from build123d import *

# Parameters (mm, degrees)
F1_DEPTH   = 25
F1_FACE_W  = 5
F1_FACE_H  = 25
F1_FACE1_W = 25
F1_FACE1_H = 25


with BuildPart() as f1:
    # F0 (on Front) → F1 (new body)
    with BuildSketch(Plane.XZ):
        Polygon((0, -93.0193822413), (0, 61.6336810916), (25, 61.6336810916), (25, -93.0193822413), (50, -93.0193822413), (50, 61.6336810916), (45, 61.6336810916), (45, -88.0193822413), (30, -88.0193822413), (30, 66.6336810916), (-5, 66.6336810916), (-5, -93.0193822413), align=None)
    extrude(amount=F1_DEPTH)

    # F1_face (on face) → F2 section 0
    with BuildSketch(Plane(origin=(47.5, -12.5, 61.6336810916), x_dir=(1, 0, 0), z_dir=(0, 0, 1))):
        Rectangle(F1_FACE_W, F1_FACE_H)
    # F1_face1 (on face) → F2 section 1
    with BuildSketch(Plane(origin=(37.5, -12.5, -93.0193822413), x_dir=(1, 0, 0), z_dir=(0, 0, -1))):
        Rectangle(F1_FACE1_W, F1_FACE1_H)
    loft()


solid = f1.part
Here's how the part is built. I have some questions about the finished solid (model axes, mm). A direction names the side the tool comes from. Coordinates: 2 decimals unless noted, no trailing zeros. Write each loop counter-clockwise with the first axis right and the second up, starting at its lowest first coordinate (ties: lowest second). Pieces come first, ordered by that corner, then holes.
1) If I drill on line 1 (X direction, y = -5.75, z = -21); line 2 (X direction, y = -23.5, z = -52); line 3 (X direction, y = -17.25, z = -84), over which ranges is the centre line in solid material (lowest first)?
Filled in:
line 1: x = -5 to 0, 25 to 30, 34.31 to 50
line 2: x = -5 to 0, 25 to 30, 30.3 to 50
line 3: x = -5 to 0, 25 to 50
2) If we section it at D-D (x = 15): List the corners of the cut face in (y, z) for me, plus the area to 3 significant figures.
Filled in:
outline: (-25, 61.63) - (0, 61.63) - (0, 66.63) - (-25, 66.63) - close
area: 125 mm2
3) If we section it at C-C (z = -37): List the corners of the cut face in (x, y) for me, plus the area to 3 significant figures.
Filled in:
outline: (-5, -25) - (0, -25) - (0, 0) - (-5, 0) - close; (25, -25) - (30, -25) - (30, 0) - (25, 0) - close; (32.24, -25) - (50, -25) - (50, 0) - (32.24, 0) - close
area: 694 mm2
4) Thinking about a two-plate mould opening in X: for faces 4 (the face through (50, -12, -17)), 5 (the face through (48, -12, 61.634)), 6 (the face through (0, -12, -17)), which applies, +X half, -X half, draft (parallel to the pull), parting line (faces both ways), or undercut?
Filled in:
face 4: +X half
face 5: draft
face 6: undercut
5) I'm going to push flat-ended pins straight in: pin 1 (1.5 mm diameter, centred on x = 1.5, y = -9, fed in from -Z); pin 2 (2.5 mm diameter, centred on x = 46.5, y = -10, fed in from +Z). Where does each tip first touch, or does it pass through?
Filled in:
pin 1: stops at z = 61.63
pin 2: stops at z = 61.63
6) If we section it at A-A (z = -65.5): List the corners of the cut face in (x, y) for me, plus the area to 3 significant figures.
Filled in:
outline: (-5, -25) - (0, -25) - (0, 0) - (-5, 0) - close; (25, -25) - (50, -25) - (50, 0) - (25, 0) - close
area: 750 mm2
7) If we section it at B-B (y = -4.25): List the corners of the cut face in (x, z) for me.
Filled in:
outline: (-5, -93.02) - (0, -93.02) - (0, 61.63) - (25, 61.63) - (25, -93.02) - (50, -93.02) - (50, 61.63) - (45, 61.63) - (30, -54.36) - (30, 66.63) - (-5, 66.63) - close
8) Which directions (+Z, -Z, +X, -X, +Y, -Y) give clear straight access to the entire face, cutting with the end or side of a thin tool? Please do faces 1 (the face through (37.395, -12.325, 2.827)), 2 (the face through (-5, -12, -12)), 3 (the face through (12, -12, 61.634)).
Filled in:
face 1: +Z, +Y, -Y
face 2: +Z, -Z, -X, +Y, -Y
face 3: -Z, +Y, -Y
